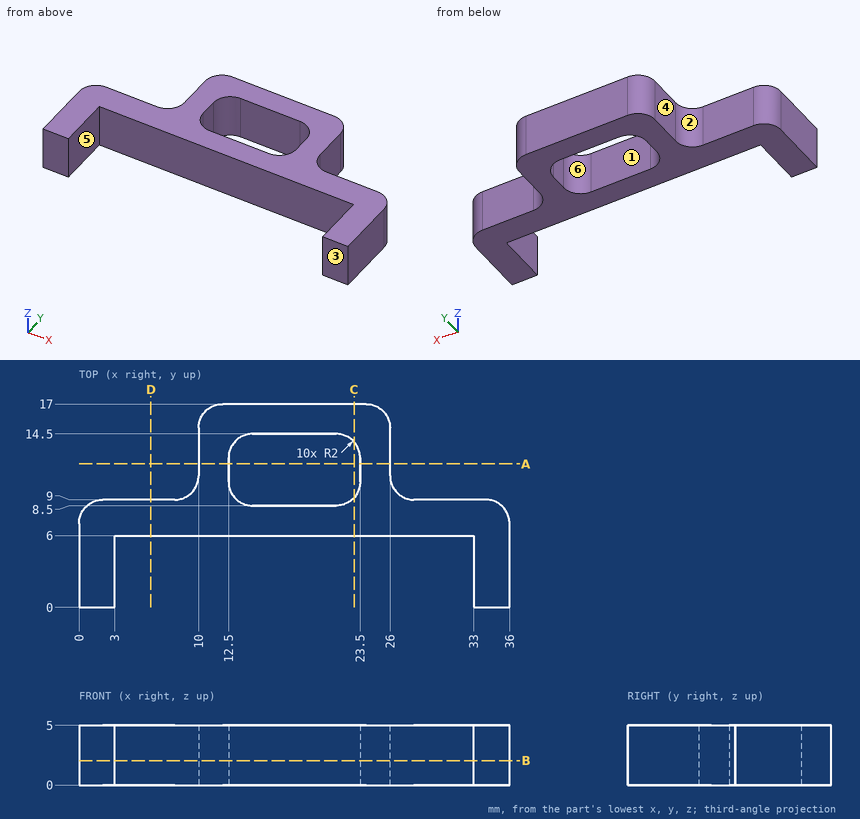
Part print with two shaded views. Sizes in mm from the minimum x, y, z corner. A direction names the side the tool comes from. Round coordinates to 2 decimals unless told otherwise and drop trailing zeros. Loops run counter-clockwise (first coordinate to the right, second up) from the corner with the lowest first, then second, coordinate; pieces in that order, holes last. Notation, with made-up numbers: M -6,18 L 38,18 A25 ccw 38,43 Z; hole C 51,-5 d6. An arc over 180 degrees is marked long. Put each result on its own line as item: value. Start each with the question number.
Item 1: 3-axis set-ups, long thin cutter, end or side, ignore diameter. For the marked faces 4, 5 and 6: which of +Z, -Z, +X, -X, +Y, -Y reach the whole face in a straight line?
Item 2: Drop flat-ended pins along their axis: P1, Ø1.5, axis at x = 5.5, z = 2.5, coming from the +Y side; P2, Ø1, axis at y = 11, z = 3.5, coming from the +X side; P3, Ø2, axis at x = 26.5, y = 14.5, coming from the -Z side; P4, Ø2.5, axis at x = 13, z = 2.5, coming from the -Y side. Give the stop position or say it passes through.
Item 3: Cut at B-B (z = 2.05). List the corners of the cut face in (x, y).
Item 4: Drill centre lines: line 1 along X through (y, z) = (12.5, 1.3); line 2 along Y through (x, z) = (21.5, 3.35); line 3 along X through (y, z) = (3.25, 2.4). Where is each one in solid material? Low to high.
Item 5: Cut at D-D (x = 6). List the corners of the cut face in (y, z), then the cut area to 3 significant figures.
Item 6: Cut at C-C (x = 23). List the corners of the cut face in (y, z).
Item 7: Mould opens along Y. For the marked faces 1, 2 and 3 say: released by +Y, released by -Y, zero draft, split by the parting line, or undercut.
Item 8: Cut at A-A (y = 12). List the corners of the cut face in (x, z).
Answer block:
1. face 4: +Z, -Z, -X, +Y
1. face 5: +Z, -Z, -Y
1. face 6: +Z, -Z
2. P1: y = 9
2. P2: x = 26.06
2. P3: z = 0
2. P4: y = 6
3. outline: M 0,0 L 3,0 L 3,6 L 33,6 L 33,0 L 36,0 L 36,7 A2 ccw 34,9 L 28,9 A2 cw 26,11 L 26,15 A2 ccw 24,17 L 12,17 A2 ccw 10,15 L 10,11 A2 cw 8,9 L 2,9 A2 ccw 0,7 Z; hole M 12.5,10.5 A2 ccw 14.5,8.5 L 21.5,8.5 A2 ccw 23.5,10.5 L 23.5,12.5 A2 ccw 21.5,14.5 L 14.5,14.5 A2 ccw 12.5,12.5 Z
4. line 1: 10 to 12.5, 23.5 to 26
4. line 2: 6 to 8.5, 14.5 to 17
4. line 3: 0 to 3, 33 to 36
5. outline: M 6,0 L 9,0 L 9,5 L 6,5 Z
5. area: 15.0 mm2
6. outline: M 6,0 L 9.18,0 L 9.18,5 L 6,5 Z; M 13.82,0 L 17,0 L 17,5 L 13.82,5 Z
7. face 1: undercut
7. face 2: released by +Y
7. face 3: released by -Y
8. outline: M 10,0 L 12.5,0 L 12.5,5 L 10,5 Z; M 23.5,0 L 26,0 L 26,5 L 23.5,5 Z
